Here's how the part is built. I have some questions about the finished solid (model axes, mm). A direction names the side the tool comes from. Give positions to 0.01 mm unless a question says otherwise; leave off trailing zeros. Loops run counter-clockwise (first coordinate to the right, second up) from the corner with the lowest first, then second, coordinate; pieces in that order, holes last. Notation, with made-up numbers: (75.5, 78) -> (116.5, 78) arc R32 cw to (116.5, 106) -> close; hole circle Ø3 at (14.25, 38). An arc over 180 degrees is marked (long way). Answer in a Markdown table with one row per item. Add a question column.
Item 1: Which directions (+Z, -Z, +X, -X, +Y, -Y) give clear straight access to the entire face, cutting with the end or side of a thin tool? Please do faces 1 (the face through (676, -1, 2.5)), 2 (the face through (700, -1, 14)).
Item 2: We'd pull the mould along Y, two halves only. Please class faces 3 (the face through (348, 40, 27)), 4 (the face through (348, -40, 27)), 5 (the face through (345, -1, 26.5)): released by +Y, released by -Y, zero draft, split by the parting line, or undercut.
Item 3: If I drill on line 1 (Y direction, x = 323.5, z = 28.35); line 2 (X direction, y = -17, z = 28.35); line 3 (Y direction, x = 670, z = 1.2), over which ranges is the centre line in solid material (lowest first)?
Item 4: If we section it at A-A (z = 17): Write out the boundary of the cut face in (x, y), then the cut area to 3 significant figures.
Item 5: If we section it at B-B (y = 28): Write out the boundary of the cut face in (x, z), then the cut area to 3 significant figures.
Item 6: For P1, Ø4, axis at x = 323.5, y = -17, coming from the -Z side (3 decimals); P2, Ø9, axis at x = 381.5, y = 17, coming from the -Z side; P3, Ø1.2, axis at y = -18, z = 2, coming from the +X side; P4, Ø1.2, axis at y = 17.5, z = 1, coming from the -X side, each with a flat end and sliding along its axis, tell me the tip position at first contact or that it passes through.
Item 7: If we section it at C-C (x = 627.5): Write out the boundary of the cut face in (y, z), then the cut area to 3 significant figures.
```python
from build123d import *

# Parameters (mm, degrees)
F1_DEPTH = 40
F4_D     = 9
F4_DEPTH = 12
F4_TIP   = 2.7038727856
F5_D     = 9
F5_DEPTH = 12
F5_TIP   = 2.7038727856
F7_D     = 7
F8_R     = 5


# Not quite as in the source:
# - a feature names something its author has since deleted; it is built from what else it names


with BuildPart() as f1:
    # F0 (on Front) → F1 (new body, symmetric)
    with BuildSketch(Plane.XZ):
        Polygon((0, 29), (0, 0), (50, 0), (50, 2.5), (2.5, 2.5), (2.5, 26.5), (697.5, 26.5), (697.5, 2.5), (650, 2.5), (650, 0), (700, 0), (700, 29), align=None)
    extrude(amount=F1_DEPTH, both=True)

    # F4 (one way)
    with BuildSketch(Plane.XY.offset(2.5)):
        with Locations((670, 0)):
            Circle(F4_D / 2)
    extrude(amount=-F4_DEPTH, mode=Mode.SUBTRACT)
    with Locations(Plane.XY.offset(2.5)):
        with Locations((670, 0)):
            with Locations((0, 0, -(F4_DEPTH + F4_TIP / 2))):  # 118° drill point
                Cone(0, F4_D / 2, F4_TIP, mode=Mode.SUBTRACT)

    # F5 (one way)
    with BuildSketch(Plane.XY.offset(2.5)):
        with Locations((30, 0)):
            Circle(F5_D / 2)
    extrude(amount=-F5_DEPTH, mode=Mode.SUBTRACT)
    with Locations(Plane.XY.offset(2.5)):
        with Locations((30, 0)):
            with Locations((0, 0, -(F5_DEPTH + F5_TIP / 2))):  # 118° drill point
                Cone(0, F5_D / 2, F5_TIP, mode=Mode.SUBTRACT)

    # F7 (through all)
    with Locations(Plane(origin=(0, 0, 26.5), x_dir=(1, 0, 0), z_dir=(0, 0, -1))):
        with Locations((381.5, -17), (323.5, -17), (323.5, 17), (381.5, 17)):
            Hole(F7_D / 2)

    # F8
    f8_edges = [f1.edges().sort_by_distance(p)[0] for p in [
        (0, 0, 29),
        (0, 0, 0),
        (700, 0, 29),
        (700, 0, 0),
        (2.5, 0, 2.5),
        (2.5, 0, 26.5),
        (697.5, 0, 2.5),
        (697.5, 0, 26.5),
    ]]
    fillet(f8_edges, radius=F8_R)


solid = f1.part
```
Recorded:
| question | item | result |
|---|---|---|
| 1 | face 1 | +Y, -Y |
| 1 | face 2 | +Z, -Z, +X, +Y, -Y |
| 2 | face 3 | released by +Y |
| 2 | face 4 | released by -Y |
| 2 | face 5 | zero draft |
| 3 | line 1 | y = -40 to -20.5, -13.5 to 13.5, 20.5 to 40 |
| 3 | line 2 | x = 2.53 to 320, 327 to 378, 385 to 697.47 |
| 3 | line 3 | y = -40 to -4.5, 4.5 to 40 |
| 4 | outline | (0, -40) -> (2.5, -40) -> (2.5, 40) -> (0, 40) -> close; (697.5, -40) -> (700, -40) -> (700, 40) -> (697.5, 40) -> close |
| 4 | area | 400 mm^2 |
| 5 | outline | (0, 5) arc R5 ccw to (5, 0) -> (50, 0) -> (50, 2.5) -> (7.5, 2.5) arc R5 cw to (2.5, 7.5) -> (2.5, 21.5) arc R5 cw to (7.5, 26.5) -> (692.5, 26.5) arc R5 cw to (697.5, 21.5) -> (697.5, 7.5) arc R5 cw to (692.5, 2.5) -> (650, 2.5) -> (650, 0) -> (695, 0) arc R5 ccw to (700, 5) -> (700, 24) arc R5 ccw to (695, 29) -> (5, 29) arc R5 ccw to (0, 24) -> close |
| 5 | area | 2,120 mm^2 |
| 6 | P1 | passes through |
| 6 | P2 | stops at z = 26.5 |
| 6 | P3 | stops at x = 699.39 |
| 6 | P4 | stops at x = 1.33 |
| 7 | outline | (-40, 26.5) -> (40, 26.5) -> (40, 29) -> (-40, 29) -> close |
| 7 | area | 200 mm^2 |
